Build history of the part. All positions in model axes, mm. A direction names the side the tool comes from. Coordinates: 2 decimals unless noted, no trailing zeros. Loops run counter-clockwise (first coordinate to the right, second up) from the corner with the lowest first, then second, coordinate; pieces in that order, holes last. Notation, with made-up numbers: (68, -27.75) -> (77, -27.75) arc R15 cw to (77, -21.75) -> close; hole circle Ø11 at (48.25, 78.5). An arc over 180 degrees is marked (long way). One line per item, written item: value. Start each with the question number.
```python
from build123d import *

# Parameters (mm, degrees)
F2_W          = 2
F2_H          = 4.9041104602
F3_DEPTH      = 6.501
F3_DEPTH_BACK = 6.501


with BuildPart() as f1:
    # F0 (on Front) → F1 (revolve)
    with BuildSketch(Plane.XZ):
        Polygon((0, 18.2320508076), (0, 0), (3, 1.7320508076), (3, 14.7320508076), (6.5, 18.2320508076), align=None)
    revolve(axis=Axis((0, 0, 9.1160254038), (0, 0, -1)))

    # F2 (on Front) → F3 (cut, two sides)
    with BuildSketch(Plane.XZ) as f3_sk:
        with Locations((0, 19.6841060377)):
            Rectangle(F2_W, F2_H)
    extrude(amount=-F3_DEPTH, mode=Mode.SUBTRACT)
    extrude(f3_sk.sketch, amount=F3_DEPTH_BACK, mode=Mode.SUBTRACT)


solid = f1.part
```
Item 1: Tool access for faces 4 (the face through (-3, 0, 8)), 5 (the face through (-3, 0, 18.232)), 6 (the face through (1, 0, 18)): list every direction of +Z, -Z, +X, -X, +Y, -Y with a clear straight run to the whole face (end or side of a thin tool).
Item 2: Band-saw the part on B-B, the plane z = 15.25. List the corners of the cut face in (x, y).
Item 3: Probe probe 1 along Y at (x, z) = (0, 8.25); probe 2 along Y at (x, z) = (-1, 4); probe 3 along Z at (x, y) = (2.5, -2.5). List the from-to ranges inside material, lowest first.
Item 4: Two-plate mould, pull along X, no slides. Class faces 1 (the face through (3, 0, 18.232)), 2 (the face through (-0.11, 0.51, 0.3)), 3 (the face through (-1, 0, 18)): +X half, -X half, draft (parallel to the pull), parting line (faces both ways), or undercut.
Item 5: Drop flat-ended pins along their axis: pin 1 Ø5 at (x, z) = (-2.5, 5) entering from +Y; pin 2 Ø3 at (y, z) = (-3, 13) entering from -X; pin 3 Ø5 at (y, z) = (3.5, 4) entering from +X. Give the stop position or say it passes through.
Item 6: Band-saw the part on A-A, the plane z = 2.25. List the corners of the cut face in (x, y), and give its area (3 significant figures).
Worked out:
1. face 4: -Z
1. face 5: +Z, +X, -X, +Y, -Y
1. face 6: +Z, +Y, -Y
2. outline: circle Ø7.04 at (0, 0)
3. probe 1: y = -3 to 3
3. probe 2: y = -2.83 to 2.83
3. probe 3: z = 15.27 to 18.23
4. face 1: draft
4. face 2: parting line
4. face 3: undercut
5. pin 1: stops at y = 3
5. pin 2: stops at x = -2.6
5. pin 3: stops at x = 2.83
6. outline: circle Ø6 at (0, 0)
6. area: 28.3 mm²
